Source: CAD feature listing. Evaluate the final solid. Frame: model axes, mm. A direction names the side the tool comes from. Give positions to 0.01 mm unless a question says otherwise; leave off trailing zeros. Order: outer loops, then holes, each group sorted by start corner. A loop starts at its lowest first (then second) coordinate and runs counter-clockwise, first axis right, second up. Notation, with made-up numbers: (17.5, -1.5) - (52.5, -1.5) arc R29 ccw to (52.5, 29.5) - close; hole circle Ø6 at (47, 31). An arc over 180 degrees is marked (long way). Use CSV: the item, a comma, the result in double quotes.
```python
from build123d import *

# Parameters (mm, degrees)
PAD007_DEPTH  = 4
SKETCH023_W   = 4
SKETCH023_H   = 10
PAD008_DEPTH  = 35
SKETCH024_R   = 1.45
HOLE005_DEPTH = 86.001
FILLET004_R   = 4
FILLET005_R   = 2


with BuildPart() as part:
    # Sketch022 (on DatumPlane) → Pad007 (new body)
    with BuildSketch(Plane(origin=(-27.5, 0, -70), x_dir=(1, 0, 0), z_dir=(0, 0, 1))):
        with BuildLine():
            Line((2.5, 164.5), (-12.5, 164.5))
            Line((-12.5, 164.5), (-12.5, 109.5))
            Line((-12.5, 109.5), (-15.499998, 109.5))
            Line((-15.499998, 109.5), (-15.499998, 94.5))
            Line((-15.499998, 94.5), (2e-06, 94.5))
            Line((2e-06, 94.5), (2e-06, 109.499996))
            Line((2e-06, 109.499996), (55.000002, 109.5))
            Line((55.000002, 109.5), (55.000002, 94.5))
            Line((55.000002, 94.5), (70.500002, 94.5))
            Line((70.500002, 94.5), (70.500002, 109.5))
            Line((70.500002, 109.5), (67.500004, 109.5))
            Line((67.500004, 109.5), (67.500004, 164.5))
            Line((67.500004, 164.5), (52.500004, 164.5))
            Line((52.500004, 164.5), (52.5, 139.499996))
            ThreePointArc((2.5, 139.5), (27.499998, 114.5), (52.5, 139.499996))
            Line((2.5, 164.5), (2.5, 139.5))
        make_face()
    extrude(amount=PAD007_DEPTH)

    # Sketch023 (on Face18 of Pad007) → Pad008 (join)
    with BuildSketch(Plane(origin=(-27.5, 0, -66), x_dir=(1, 0, 0), z_dir=(0, 0, 1))):
        with Locations((-5.499998, 99.5)):
            Rectangle(SKETCH023_W, SKETCH023_H)
        with Locations((60.500002, 99.5)):
            Rectangle(SKETCH023_W, SKETCH023_H)
        with Locations((68.500002, 99.5)):
            Rectangle(SKETCH023_W, SKETCH023_H)
        with Locations((-13.499998, 99.5)):
            Rectangle(SKETCH023_W, SKETCH023_H)
    extrude(amount=PAD008_DEPTH)

    # Sketch024 (on Face32 of Pad008) → Hole005 (cut, through all)
    with BuildSketch(Plane(origin=(43.000002, 0, -70), x_dir=(0, 1, 0), z_dir=(1, 0, 0))):
        with Locations((99.5, 34)):
            Circle(SKETCH024_R)
        with Locations((99.5, 28)):
            Circle(SKETCH024_R)
    extrude(amount=-HOLE005_DEPTH, mode=Mode.SUBTRACT)

    # Fillet004
    fillet004_edges = [part.edges().sort_by_distance(p)[0] for p in [
        (-40.999998, 94.5, -31),
        (-40.999998, 104.5, -31),
        (-32.999998, 104.5, -31),
        (-32.999998, 94.5, -31),
        (33.000002, 94.5, -31),
        (33.000002, 104.5, -31),
        (41.000002, 104.5, -31),
        (41.000002, 94.5, -31),
    ]]
    fillet(fillet004_edges, radius=FILLET004_R)

    # Fillet005
    fillet005_edges = [part.edges().sort_by_distance(p)[0] for p in [
        (43.000002, 109.5, -68),
        (40.000004, 164.5, -68),
        (25.000004, 164.5, -68),
        (-25, 164.5, -68),
        (-40, 164.5, -68),
        (-42.999998, 109.5, -68),
    ]]
    fillet(fillet005_edges, radius=FILLET005_R)


with BuildPart() as part_1:
    # Body002 placement: moved
    add(part.part.moved(Location((0.099998, -1.370226, -11.596799))))


solid = part_1.part
```
Item 1: Section D-D on x = 30. Return the cut outline in (y, z), then the cut area to 3 significant figures.
Filled in:
outline,"(93.13, -81.6) - (163.13, -81.6) - (163.13, -77.6) - (93.13, -77.6) - close"
area,"280 mm2"
Item 2: Material intervals for line 1 (X direction, y = 102, z = -71.5); line 2 (X direction, y = 110, z = -79); line 3 (Z direction, x = -33, y = 133), sorted ascending. Write a range as from..to.
Filled in:
line 1,"x = -42.9..-38.9, -34.9..-30.9, 31.1..35.1, 39.1..43.1"
line 2,"x = -39.9..40.1"
line 3,"z = -81.6..-77.6"
Item 3: Mould query, pull axis X, two halves, no side actions, for faces 1 (the flat face through (33, 163.13, -80)), 2 (the cylindrical face through (-42.33, 107.53, -79.57)), 3 (the cylindrical face through (-0.45, 113.136, -79.625)), 4 (the cylindrical face through (39.5, 162.56, -79.57)). Classes: released by +X, released by -X, zero draft, split by the parting line, or undercut.
Filled in:
face 1,"zero draft"
face 2,"released by -X"
face 3,"undercut"
face 4,"released by +X"
Item 4: Section B-B on z = -71. Return the cut outline in (x, y).
Filled in:
outline,"(-42.9, 93.13) - (-38.9, 93.13) - (-38.9, 103.13) - (-42.9, 103.13) - close; (-34.9, 93.13) - (-30.9, 93.13) - (-30.9, 103.13) - (-34.9, 103.13) - close; (31.1, 93.13) - (35.1, 93.13) - (35.1, 103.13) - (31.1, 103.13) - close; (39.1, 93.13) - (43.1, 93.13) - (43.1, 103.13) - (39.1, 103.13) - close"
Item 5: First-contact query: pin 1 (8 mm diameter, centred on y = 125, z = -77, fed in from -X); pin 2 (3 mm diameter, centred on x = 21.5, y = 134.5, fed in from +Z); pin 3 (4 mm diameter, centred on x = 33.5, y = 130.5, fed in from +Z); pin 4 (3 mm diameter, centred on x = 6, z = -79.5, fed in from -Y). Flat tips, straight axial feed; report the tip coordinate or a pass-through.
Filled in:
pin 1,"stops at x = -39.9"
pin 2,"passes through"
pin 3,"stops at z = -77.6"
pin 4,"stops at y = 108.13"
Item 6: Section C-C on y = 121. Return the cut outline in (x, z), then the cut area to 3 significant figures.
Filled in:
outline,"(-39.9, -81.6) - (-18.11, -81.6) - (-18.11, -77.6) - (-39.9, -77.6) - close; (18.31, -81.6) - (40.1, -81.6) - (40.1, -77.6) - (18.31, -77.6) - close"
area,"174 mm2"
Item 7: Section A-A on y = 143. Return the cut outline in (x, z).
Filled in:
outline,"(-39.9, -81.6) - (-24.9, -81.6) - (-24.9, -77.6) - (-39.9, -77.6) - close; (25.1, -81.6) - (40.1, -81.6) - (40.1, -77.6) - (25.1, -77.6) - close"
Item 8: Set-up query: faces 5 (the flat face through (-33, 103.13, -62)), 6 (the cylindrical face through (25.67, 162.53, -79.57)), 7 (the flat face through (31.1, 98, -60)). Return all of +Z, -Z, +X, -X, +Y, -Y with unobstructed straight access to the full face (end or side cutting, diameter ignored); none if empty.
Filled in:
face 5,"+Z, +X, -X, +Y"
face 6,"+Z, -Z, +Y"
face 7,"+Z, +Y, -Y"
